Geometry: final body of the model. Coordinates: model frame, mm. A direction names the side the tool comes from. Coordinates: 2 decimals unless noted, no trailing zeros. Write each loop counter-clockwise with the first axis right and the second up, starting at its lowest first coordinate (ties: lowest second). Pieces come first, ordered by that corner, then holes. Notation, with made-up numbers: (-37.5, -4) - (-27.5, -4) arc R21 ccw to (-27.5, 22) - close; hole circle Ø3 at (53, -25.75). An arc over 180 degrees is marked (long way). Put each result on its own line as item: value.
```python
from build123d import *

# Parameters (mm, degrees)
SKETCH1_W           = 3
SKETCH1_H           = 24
BOSS_EXTRUDE1_DEPTH = 23
SKETCH2_W           = 6
SKETCH2_H           = 24
BOSS_EXTRUDE2_DEPTH = 2
SKETCH3_W           = 22
SKETCH3_H           = 9
CUT_EXTRUDE1_DEPTH  = 1
SKETCH4_W           = 3
SKETCH4_H           = 24
BOSS_EXTRUDE3_DEPTH = 2


with BuildPart() as part:
    # Sketch1 → Boss-Extrude1 (new body)
    with BuildSketch(Plane(origin=(0, 0, 0), x_dir=(1, 0, 0), z_dir=(0, 1, 0))):
        with Locations((1.5, 12)):
            Rectangle(SKETCH1_W, SKETCH1_H)
    extrude(amount=BOSS_EXTRUDE1_DEPTH)

    # Sketch2 → Boss-Extrude2 (add)
    with BuildSketch(Plane(origin=(0, 23, 0), x_dir=(1, 0, 0), z_dir=(0, 1, 0))):
        with Locations((0, 12)):
            Rectangle(SKETCH2_W, SKETCH2_H)
    extrude(amount=BOSS_EXTRUDE2_DEPTH)

    # Sketch3 → Cut-Extrude1 (cut)
    with BuildSketch(Plane.ZY):
        with Locations((-12, 16.5)):
            Rectangle(SKETCH3_W, SKETCH3_H)
    extrude(amount=-CUT_EXTRUDE1_DEPTH, mode=Mode.SUBTRACT)

    # Sketch4 → Boss-Extrude3 (add)
    with BuildSketch(Plane.XZ):
        with Locations((1.5, -12)):
            Rectangle(SKETCH4_W, SKETCH4_H)
    extrude(amount=BOSS_EXTRUDE3_DEPTH)


solid = part.part
```
1. Pin query (flat end, axial travel): pin 1 Ø3 at (y, z) = (7, -5.5) entering from -X; pin 2 Ø2.5 at (y, z) = (18.5, -10) entering from -X; pin 3 Ø0.9 at (x, z) = (-2, -6.5) entering from -Y. Return the tip coordinate at first contact, or that it passes through.
Answer below:
pin 1: stops at x = 0
pin 2: stops at x = 1
pin 3: stops at y = 23
2. Mould query, pull axis Z, two halves, no side actions, for faces 4 (the flat face through (0.5, 12, -12.2)), 5 (the flat face through (3, 12, -12)), 6 (the flat face through (1, 12, -24)). Classes: +Z half, -Z half, draft (parallel to the pull), parting line (faces both ways), or undercut.
Answer below:
face 4: undercut
face 5: draft
face 6: -Z half
3. Section query B-B (y = 14.5). Return loops of the section in (x, z).
Answer below:
outline: (0, -24) - (3, -24) - (3, 0) - (0, 0) - (0, -1) - (1, -1) - (1, -23) - (0, -23) - close
4. Set-up query: faces 1 (the flat face through (0.5, 21, -12.2)), 2 (the flat face through (1, -2, -12)), 3 (the flat face through (-2, 23, -12)). Return all of +Z, -Z, +X, -X, +Y, -Y with unobstructed straight access to the full face (end or side cutting, diameter ignored); none if empty.
Answer below:
face 1: -X
face 2: +Z, -Z, +X, -X, -Y
face 3: +Z, -Z, -X, -Y
5. Section query A-A (z = -15). Return loops of the section in (x, y), then the cut area to 3 significant figures.
Answer below:
outline: (-3, 23) - (0, 23) - (0, 21) - (1, 21) - (1, 12) - (0, 12) - (0, -2) - (3, -2) - (3, 25) - (-3, 25) - close
area: 78.0 mm²
6. Section query C-C (x = -0.4). Return loops of the section in (y, z).
Answer below:
outline: (23, -24) - (25, -24) - (25, 0) - (23, 0) - close
7. Ray query, probe 1 along Z at (x, y) = (0.45, 18.25); probe 2 along Y at (x, z) = (0.15, -15.75); probe 3 along X at (y, z) = (14, -22). Return the intervals inside material, ascending. Write a range as from..to.
Answer below:
probe 1: z = -24..-23, -1..0
probe 2: y = -2..12, 21..25
probe 3: x = 1..3
8. Section query D-D (y = 11.25). Return loops of the section in (x, z).
Answer below:
outline: (0, -24) - (3, -24) - (3, 0) - (0, 0) - close
